```python
from build123d import *

# Parameters (mm, degrees)
F0_R     = 12.7
F1_DEPTH = 7
F2_R     = 9
F3_DEPTH = 10
F4_R     = 6
F5_DEPTH = 17.001
F7_D     = 5
F7_DEPTH = 12.701


with BuildPart() as f1:
    # F0 (on Front) → F1 (new body)
    with BuildSketch(Plane.XZ):
        Circle(F0_R)
    extrude(amount=F1_DEPTH)

    # F2 (on Front) → F3 (join)
    with BuildSketch(Plane.XZ):
        Circle(F2_R)
    extrude(amount=-F3_DEPTH)

    # F4 (on face) → F5 (cut, through all)
    with BuildSketch(Plane.XZ.offset(7)):
        Circle(F4_R)
    extrude(amount=-F5_DEPTH, mode=Mode.SUBTRACT)

    # F7 (through all, one way)
    with BuildSketch(Plane.XY):
        with Locations((0, 5)):
            Circle(F7_D / 2)
    extrude(amount=-F7_DEPTH, mode=Mode.SUBTRACT)


solid = f1.part
```
Part model, mm, in its own coordinate system. A direction names the side the tool comes from. Coordinates: 2 decimals unless noted, no trailing zeros. Loops run counter-clockwise (first coordinate to the right, second up) from the corner with the lowest first, then second, coordinate; pieces in that order, holes last. Notation, with made-up numbers: (45, 51) - (52, 51) arc R11 cw to (52, 59) - close; hole circle Ø10 at (38.5, -1.5). An arc over 180 degrees is marked (long way). Write item = value, one per line. Start each with the question number.
Item 1: Mould opens along X. For faces 3 (the flat face through (2, 10, -6)), 4 (the cylindrical face through (1.34, 7.11, -7.21)), 5 (the cylindrical face through (-2.75, -3.45, -12.4)) say: released by +X, released by -X, zero draft, split by the parting line, or undercut.
Item 2: Flat gauge pins, fed straight in: pin 1 Ø1.5 at (y, z) = (5.5, 3) entering from +X; pin 2 Ø1 at (y, z) = (4, -3) entering from -X; pin 3 Ø3 at (x, y) = (0, 5) entering from -Z. Where does each tip first touch, or does it go through?
Item 3: Cut at C-C, the plane y = -4.5. Give the cut face in (x, z), and give its area (3 significant figures).
Item 4: Wall check: L1, parallel to Z at x = 0, y = -2.5; L2, parallel to Y at x = 10.5, z = -5.5; L3, parallel to Y at x = 0, z = -7.95. Give the ranges that are in metal, low to high. Write a range as from..to.
Item 5: Cut at A-A, the plane x = 0. Give the cut face in (y, z).
Item 6: 3-axis set-ups, long thin cutter, end or side, ignore diameter. For faces 1 (the cylindrical face through (-1.172, 4.93, 8.923)), 2 (the cylindrical face through (-0.78, 1.38, 5.95)): which of +Z, -Z, +X, -X, +Y, -Y reach the whole face in a straight line?
Item 7: Cut at B-B, the plane z = 0. Give the cut face in (x, y).
Item 8: Cut at D-D, the plane x = -5.25. Give the cut face in (y, z).
The answers:
q1.face_3 = zero draft
q1.face_4 = undercut
q1.face_5 = split by the parting line
q2.pin_1 = 8.71
q2.pin_2 = -8.65
q2.pin_3 = 5.81
q3.outline = circle Ø25.4 at (0, 0); hole circle Ø12 at (0, 0)
q3.area = 394 mm2
q4.L1 = -12.7..-6, 6..12.7
q4.L2 = -7..0
q4.L3 = -7..2.5, 7.5..10
q5.outline = (-7, -12.7) - (0, -12.7) - (0, -9) - (2.5, -9) - (2.5, -6) - (-7, -6) - close; (-7, 6) - (10, 6) - (10, 9) - (0, 9) - (0, 12.7) - (-7, 12.7) - close; (7.5, -9) - (10, -9) - (10, -6) - (7.5, -6) - close
q6.face_1 = +Y
q6.face_2 = +Y, -Y
q7.outline = (-12.7, -7) - (-6, -7) - (-6, 10) - (-9, 10) - (-9, 0) - (-12.7, 0) - close; (6, -7) - (12.7, -7) - (12.7, 0) - (9, 0) - (9, 10) - (6, 10) - close
q8.outline = (-7, -11.56) - (0, -11.56) - (0, -7.31) - (10, -7.31) - (10, -2.9) - (-7, -2.9) - close; (-7, 2.9) - (10, 2.9) - (10, 7.31) - (0, 7.31) - (0, 11.56) - (-7, 11.56) - close
